The listing builds one solid part. Answer for the finished solid, in the listing's coordinates (mm). Face numbers are marked on the shaded views. A direction names the side the tool comes from. Coordinates: 2 decimals unless noted, no trailing zeros. Order: outer loops, then holes, each group sorted by start corner. A loop starts at its lowest first (then second) coordinate and runs counter-clockwise, first axis right, second up. Notation, with made-up numbers: (62.5, -5.5) -> (106.5, -5.5) arc R37 cw to (106.5, 32.5) -> close; hole circle Ø8 at (58, 8). An arc over 180 degrees is marked (long way). Answer in a Markdown table with one row per item.
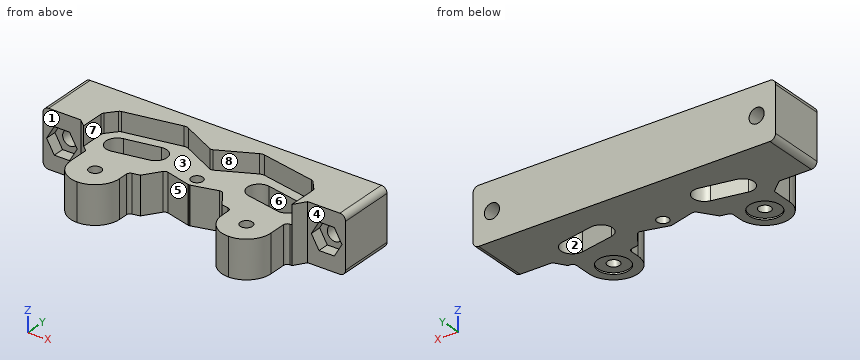
```python
from build123d import *

# Parameters (mm, degrees)
BOSS_EXTRUDE1_DEPTH = 15
CUT_EXTRUDE7_DEPTH  = 5
CUT_EXTRUDE8_DEPTH  = 35
SKETCH3_R           = 1.55
CUT_EXTRUDE10_DEPTH = 32
SKETCH10_R          = 1.6
CUT_EXTRUDE11_DEPTH = 32
SKETCH11_R          = 4.1
CUT_EXTRUDE12_DEPTH = 0.4
CUT_EXTRUDE13_DEPTH = 32
SKETCH14_R          = 2
CUT_EXTRUDE14_DEPTH = 22
CUT_EXTRUDE15_DEPTH = 3
SKETCH16_W          = 38
SKETCH16_H          = 15
CUT_EXTRUDE16_DEPTH = 20
CUT_EXTRUDE17_DEPTH = 20


with BuildPart() as part:
    # Sketch1 → Boss-Extrude1 (new body)
    with BuildSketch(Plane.XY):
        Polygon((0, 0), (48, 0), (48, -15), (108, -15), (108, 0), (156, 0), (156, 15), (0, 15), align=None)
    extrude(amount=BOSS_EXTRUDE1_DEPTH)

    # Sketch2 → Cut-Extrude7 (cut)
    with BuildSketch(Plane.XY.offset(15)):
        with BuildLine():
            Line((77.552786405, 6.223606798), (68.60756702, 10.69621649))
            ThreePointArc((68.60756702, 10.69621649), (67.984760984, 10.888831752), (67.333096015, 10.870921809))
            Line((67.333096015, 10.870921809), (52.849985824, 8.067739192))
            ThreePointArc((52.849985824, 8.067739192), (52.531353266, 7.946930093), (52.271786451, 7.726143741))
            Line((52.271786451, 7.726143741), (50.23177872, 5.278134464))
            ThreePointArc((50.23177872, 5.278134464), (50.059728422, 4.978375329), (50, 4.637950065))
            Line((50, 4.637950065), (50, -15))
            Line((50, -15), (106, -15))
            Line((106, -15), (106, 4.637950065))
            ThreePointArc((106, 4.637950065), (105.940271578, 4.978375329), (105.76822128, 5.278134464))
            Line((105.76822128, 5.278134464), (103.728213549, 7.726143741))
            ThreePointArc((103.728213549, 7.726143741), (103.468646734, 7.946930093), (103.150014176, 8.067739192))
            Line((103.150014176, 8.067739192), (88.666903985, 10.870921809))
            ThreePointArc((88.666903985, 10.870921809), (88.015239016, 10.888831752), (87.39243298, 10.69621649))
            Line((87.39243298, 10.69621649), (78.447213595, 6.223606798))
            ThreePointArc((78.447213595, 6.223606798), (78, 6.118033989), (77.552786405, 6.223606798))
        make_face()
    extrude(amount=-CUT_EXTRUDE7_DEPTH, mode=Mode.SUBTRACT)

    # Sketch4 → Cut-Extrude8 (cut)
    with BuildSketch(Plane.XY.offset(15)):
        with BuildLine():
            Line((78.257662651, -1.93128996), (78, -1.960923359))
            Line((78, -1.960923359), (77.742337349, -1.93128996))
            Line((77.742337349, -1.93128996), (71.175803726, -0.180214327))
            ThreePointArc((71.175803726, -0.180214327), (70.575493167, -0.206985371), (70.098909155, -0.572986922))
            Line((70.098909155, -0.572986922), (67.200935386, -4.712949448))
            ThreePointArc((67.200935386, -4.712949448), (67.05739096, -5.016112502), (67.022171235, -5.349687697))
            Line((67.022171235, -5.349687697), (67.574638514, -14.063275904))
            ThreePointArc((67.574638514, -14.063275904), (67.888264768, -14.729135071), (68.572634586, -15))
            Line((68.572634586, -15), (87.427365414, -15))
            ThreePointArc((87.427365414, -15), (88.111735232, -14.729135071), (88.425361486, -14.063275904))
            Line((88.425361486, -14.063275904), (88.977828765, -5.349687697))
            ThreePointArc((88.977828765, -5.349687697), (88.94260904, -5.016112502), (88.799064614, -4.712949448))
            Line((88.799064614, -4.712949448), (85.901090845, -0.572986922))
            ThreePointArc((85.901090845, -0.572986922), (85.424506833, -0.206985371), (84.824196274, -0.180214327))
            Line((84.824196274, -0.180214327), (78.257662651, -1.93128996))
        make_face()
    extrude(amount=-CUT_EXTRUDE8_DEPTH, mode=Mode.SUBTRACT)

    # Sketch3 → Cut-Extrude10 (cut)
    with BuildSketch(Plane.XY.offset(15)):
        with Locations((78, 1)):
            Circle(SKETCH3_R)
    extrude(amount=-CUT_EXTRUDE10_DEPTH, mode=Mode.SUBTRACT)

    # Sketch10 → Cut-Extrude11 (cut)
    with BuildSketch(Plane.XY.offset(10)):
        with Locations((98, -8.5)):
            Circle(SKETCH10_R)
        with Locations((58, -8.5)):
            Circle(SKETCH10_R)
        with BuildLine():
            Line((54.92993428, 5.92391415), (63.765952936, 7.634111309))
            ThreePointArc((63.765952936, 7.634111309), (67.281358207, 5.258837477), (64.906084375, 1.743432206))
            Line((64.906084375, 1.743432206), (56.07006572, 0.033235047))
            ThreePointArc((56.07006572, 0.033235047), (52.554660448, 2.408508879), (54.92993428, 5.92391415))
        make_face()
        with BuildLine():
            Line((101.07006572, 5.92391415), (92.234047064, 7.634111309))
            ThreePointArc((92.234047064, 7.634111309), (88.718641793, 5.258837477), (91.093915625, 1.743432206))
            Line((91.093915625, 1.743432206), (99.92993428, 0.033235047))
            ThreePointArc((99.92993428, 0.033235047), (103.445339552, 2.408508879), (101.07006572, 5.92391415))
        make_face()
    extrude(amount=-CUT_EXTRUDE11_DEPTH, mode=Mode.SUBTRACT)

    # Sketch11 → Cut-Extrude12 (cut)
    with BuildSketch(Plane(origin=(0, 0, 0), x_dir=(-1, 0, 0), z_dir=(0, 0, -1))):
        with Locations((-58, -8.5)):
            Circle(SKETCH11_R)
        with Locations((-98, -8.5)):
            Circle(SKETCH11_R)
    extrude(amount=-CUT_EXTRUDE12_DEPTH, mode=Mode.SUBTRACT)

    # Sketch13 → Cut-Extrude13 (cut)
    with BuildSketch(Plane(origin=(0, 0, 0), x_dir=(-1, 0, 0), z_dir=(0, 0, -1))):
        with BuildLine():
            Line((-108, -15), (-98, -15))
            ThreePointArc((-98, -15), (-102.596194078, -13.096194078), (-104.5, -8.5))
            Line((-104.5, -8.5), (-104.5, -4))
            ThreePointArc((-104.5, -4), (-104.792893219, -3.292893219), (-105.5, -3))
            Line((-105.5, -3), (-106, -3))
            Line((-106, -3), (-108, 0))
            Line((-108, 0), (-108, -15))
        make_face()
        with BuildLine():
            Line((-91.5, -6.096383305), (-91.5, -8.5))
            ThreePointArc((-91.5, -8.5), (-93.403805922, -13.096194078), (-98, -15))
            Line((-98, -15), (-87.427365414, -15))
            Line((-87.427365414, -15), (-88.799064614, -4.712949448))
            Line((-88.799064614, -4.712949448), (-90.707690196, -5.11818865))
            ThreePointArc((-90.707690196, -5.11818865), (-91.277074706, -5.46697493), (-91.5, -6.096383305))
        make_face()
        with BuildLine():
            ThreePointArc((-51.5, -8.5), (-53.403805922, -13.096194078), (-58, -15))
            Line((-58, -15), (-48, -15))
            Line((-48, -15), (-48, 0))
            Line((-48, 0), (-51.5, -3))
            Line((-51.5, -3), (-51.5, -8.5))
        make_face()
        with BuildLine():
            Line((-67.200935386, -4.712949448), (-68.572634586, -15))
            Line((-68.572634586, -15), (-58, -15))
            ThreePointArc((-58, -15), (-62.596194078, -13.096194078), (-64.5, -8.5))
            Line((-64.5, -8.5), (-64.5, -6.096383305))
            ThreePointArc((-64.5, -6.096383305), (-64.722925294, -5.46697493), (-65.292309804, -5.11818865))
            Line((-65.292309804, -5.11818865), (-67.200935386, -4.712949448))
        make_face()
    extrude(amount=-CUT_EXTRUDE13_DEPTH, mode=Mode.SUBTRACT)

    # Sketch14 → Cut-Extrude14 (cut)
    with BuildSketch(Plane(origin=(0, 15, 0), x_dir=(1, 0, 0), z_dir=(0, 1, 0))):
        with Locations((113, -7.5)):
            Circle(SKETCH14_R)
        with Locations((43, -7.5)):
            Circle(SKETCH14_R)
    extrude(amount=-CUT_EXTRUDE14_DEPTH, mode=Mode.SUBTRACT)

    # Sketch15 → Cut-Extrude15 (cut)
    with BuildSketch(Plane.XZ):
        Polygon((117.041451884, 7.5), (115.020725942, 11), (110.979274058, 11), (108.958548116, 7.5), (110.979274058, 4), (115.020725942, 4), align=None)
        Polygon((38.958548116, 7.5), (40.979274058, 4), (45.020725942, 4), (47.041451884, 7.5), (45.020725942, 11), (40.979274058, 11), align=None)
    extrude(amount=-CUT_EXTRUDE15_DEPTH, mode=Mode.SUBTRACT)

    # Sketch16 → Cut-Extrude16 (cut)
    with BuildSketch(Plane(origin=(0, 15, 0), x_dir=(1, 0, 0), z_dir=(0, 1, 0))):
        with Locations((137, -7.5)):
            Rectangle(SKETCH16_W, SKETCH16_H)
        with Locations((19, -7.5)):
            Rectangle(SKETCH16_W, SKETCH16_H)
    extrude(amount=-CUT_EXTRUDE16_DEPTH, mode=Mode.SUBTRACT)

    # Sketch17 → Cut-Extrude17 (cut)
    with BuildSketch(Plane(origin=(0, 15, 0), x_dir=(1, 0, 0), z_dir=(0, 1, 0))):
        with BuildLine():
            Line((118, -13.5), (118, -15))
            Line((118, -15), (116.5, -15))
            ThreePointArc((116.5, -15), (117.560660172, -14.560660172), (118, -13.5))
        make_face()
        with BuildLine():
            Line((116.5, 0), (118, 0))
            Line((118, 0), (118, -1.5))
            ThreePointArc((118, -1.5), (117.560660172, -0.439339828), (116.5, 0))
        make_face()
        with BuildLine():
            Line((39.5, 0), (38, 0))
            Line((38, 0), (38, -1.5))
            ThreePointArc((38, -1.5), (38.439339828, -0.439339828), (39.5, 0))
        make_face()
        with BuildLine():
            Line((39.5, -15), (38, -15))
            Line((38, -15), (38, -13.5))
            ThreePointArc((38, -13.5), (38.439339828, -14.560660172), (39.5, -15))
        make_face()
    extrude(amount=-CUT_EXTRUDE17_DEPTH, mode=Mode.SUBTRACT)


solid = part.part
```
(1) Flat-ended cylindrical pins translate along their axes: pin 1 (5 mm diameter, centred on x = 78, y = 1, fed in from +Z); pin 2 (2.5 mm diameter, centred on x = 99, y = -7.5, fed in from -Z); pin 3 (6 mm diameter, centred on y = -11.5, z = 9, fed in from +X); pin 4 (1.9 mm diameter, centred on x = 58, y = -8.5, fed in from -Z). Find the tip coordinate at first contact, or state that the pin passes through.
Check values:
| item | result |
|---|---|
| pin 1 | z = 10 |
| pin 2 | z = 0.4 |
| pin 3 | x = 104.5 |
| pin 4 | through |
(2) A cutting plane is placed at B-B, the plane y = 9. Determine the outline of the cut face in (x, z).
Check values:
| item | result |
|---|---|
| outline | (38, 1.5) arc R1.5 ccw to (39.5, 0) -> (116.5, 0) arc R1.5 ccw to (118, 1.5) -> (118, 13.5) arc R1.5 ccw to (116.5, 15) -> (98.33, 15) -> (98.33, 10) -> (84, 10) -> (84, 15) -> (72, 15) -> (72, 10) -> (57.67, 10) -> (57.67, 15) -> (39.5, 15) arc R1.5 ccw to (38, 13.5) -> close; hole circle Ø4 at (43, 7.5); hole circle Ø4 at (113, 7.5) |
(3) A cutting plane is placed at D-D, the plane x = 112.5. Determine the outline of the cut face in (y, z).
Check values:
| item | result |
|---|---|
| outline | (0, 0) -> (15, 0) -> (15, 5.56) -> (3, 5.56) -> (3, 4) -> (0, 4) -> close; (0, 11) -> (3, 11) -> (3, 9.44) -> (15, 9.44) -> (15, 15) -> (0, 15) -> close |
(4) A cutting plane is placed at C-C, the plane z = 12.5. Determine the outline of the cut face in (x, y).
Check values:
| item | result |
|---|---|
| outline | (38, 0) -> (48, 0) -> (50, -1.71) -> (50, 4.64) arc R1 cw to (50.23, 5.28) -> (52.27, 7.73) arc R1 cw to (52.85, 8.07) -> (67.33, 10.87) arc R2 cw to (68.61, 10.7) -> (77.55, 6.22) arc R1 ccw to (78.45, 6.22) -> (87.39, 10.7) arc R2 cw to (88.67, 10.87) -> (103.15, 8.07) arc R1 cw to (103.73, 7.73) -> (105.77, 5.28) arc R1 cw to (106, 4.64) -> (106, -3) -> (108, 0) -> (118, 0) -> (118, 15) -> (38, 15) -> close |
(5) Find the intervals of material crossed by line 1 along X through (y, z) = (4.5, 13.5); line 2 along Z through (x, y) = (43, 8.5); line 3 along X through (y, z) = (5.5, 3.5), in increasing order. Write a range as from..to.
Check values:
| item | result |
|---|---|
| line 1 | 38..50, 106..118 |
| line 2 | 0..5.5, 9.5..15 |
| line 3 | 38..53.87, 67.22..88.78, 102.13..118 |
(6) Which of the six approach directions +Z, -Z, +X, -X, +Y, -Y give full straight-line access (tool end or side, diameter ignored) to the marked faces 1, 2, 3, 4 and 5?
Check values:
| item | result |
|---|---|
| face 1 | +Z, -Z, -X, -Y |
| face 2 | +Z, -Z |
| face 3 | +Z, -Y |
| face 4 | +Z, -Z, +X, -Y |
| face 5 | +Z, -Z, -Y |
(7) For a pull along Y with two mould halves and no side action, classify the marked faces 6, 7 and 8 as released by +Y, released by -Y, zero draft, split by the parting line, or undercut.
Check values:
| item | result |
|---|---|
| face 6 | undercut |
| face 7 | zero draft |
| face 8 | released by -Y |
(8) A cutting plane is placed at A-A, the plane x = 43. Determine the outline of the cut face in (y, z).
Check values:
| item | result |
|---|---|
| outline | (0, 0) -> (15, 0) -> (15, 5.5) -> (3, 5.5) -> (3, 4) -> (0, 4) -> close; (0, 11) -> (3, 11) -> (3, 9.5) -> (15, 9.5) -> (15, 15) -> (0, 15) -> close |
